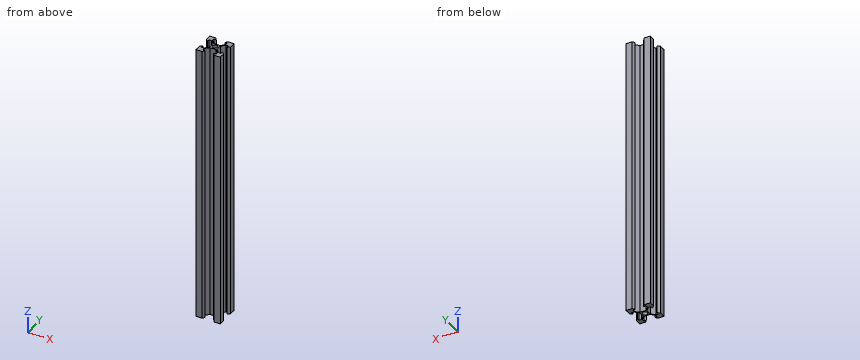
Autodesk Inventor part; units mm, degrees
ref_plane "YZ Plane" through (0, 0, 0) normal (1, 0, 0) x (0, 1, 0)
ref_plane "XZ Plane" through (0, 0, 0) normal (0, 1, 0) x (-1, 0, 0)
ref_plane "XY Plane" through (0, 0, 0) normal (0, 0, 1) x (1, 0, 0)
sketch "Sketch1" plane through (0, 0, 0) normal (0, 0, 1) x (1, 0, 0)
  line L0 (-5, 10) -> (-3.5, 8)
  line L1 (-3.5, 8) -> (-5.5, 8)
  line L2 (5.5, 8) -> (3.5, 8)
  line L3 (3.5, 8) -> (5, 10)
  line L4 (-5.5, 8) -> (-5.5, 6)
  line L5 (5.5, 8) -> (5.5, 6)
  line L6 (-5.5, 6) -> (-2.5, 3)
  line L7 (5.5, 6) -> (2.5, 3)
  line L8 (-2.5, 3) -> (2.5, 3)
  line L9 (-10, 10) -> (-5, 10)
  line L10 (5, 10) -> (10, 10)
  line L11 (3, 2.5) -> (3, -2.5)
  line L12 (3, -2.5) -> (6, -5.5)
  line L13 (6, -5.5) -> (8, -5.5)
  line L14 (8, -5.5) -> (8, -3.5)
  line L15 (8, -3.5) -> (10, -5)
  line L16 (3, 2.5) -> (6, 5.5)
  line L17 (6, 5.5) -> (8, 5.5)
  line L18 (8, 5.5) -> (8, 3.5)
  line L19 (8, 3.5) -> (10, 5)
  line L20 (10, 10) -> (10, 5)
  line L21 (10, -5) -> (10, -10)
  line L22 (-10, 5) -> (-8, 3.5)
  line L23 (-8, 3.5) -> (-8, 5.5)
  line L24 (-8, -5.5) -> (-8, -3.5)
  line L25 (-8, -3.5) -> (-10, -5)
  line L26 (-8, 5.5) -> (-6, 5.5)
  line L27 (-8, -5.5) -> (-6, -5.5)
  line L28 (-6, 5.5) -> (-3, 2.5)
  line L29 (-6, -5.5) -> (-3, -2.5)
  line L30 (-3, 2.5) -> (-3, -2.5)
  line L31 (-10, 10) -> (-10, 5)
  line L32 (-10, -5) -> (-10, -10)
  line L33 (-2.5, -3) -> (2.5, -3)
  line L34 (2.5, -3) -> (5.5, -6)
  line L35 (5.5, -6) -> (5.5, -8)
  line L36 (5.5, -8) -> (3.5, -8)
  line L37 (3.5, -8) -> (5, -10)
  line L38 (-2.5, -3) -> (-5.5, -6)
  line L39 (-5.5, -6) -> (-5.5, -8)
  line L40 (-5.5, -8) -> (-3.5, -8)
  line L41 (-3.5, -8) -> (-5, -10)
  line L42 (-10, -10) -> (-5, -10)
  line L43 (5, -10) -> (10, -10)
  point P0 (0, 0)
  point P1 (0, 0)
  point P2 (0, 0)
  dimension "d0" = 20
  dimension "d1" = 20
  dimension "d3" = 2
  dimension "d4" = 2
  dimension "d6" = 1.5
  dimension "d7" = 2
  dimension "d8" = 2
  dimension "d9" = 3
  dimension "d11" = 3
  dimension "d12" = 3
  dimension "d13" = 5
  dimension "d22" = 5
  dimension "d24" = 3
  dimension "d25" = 3
  dimension "d26" = 2
  dimension "d27" = 5
  dimension "d28" = 2
  dimension "d29" = 2
  dimension "d30" = 1.5
  dimension "d31" = 3
  dimension "d32" = 5
  dimension "d33" = 5
  dimension "d35" = 5
  dimension "d36" = 5
  dimension "d37" = 5
  dimension "d38" = 5
  dimension "d40" = 3
  dimension "d41" = 3
  dimension "d42" = 2
  dimension "d43" = 2
  dimension "d48" = 3
  dimension "d49" = 3
  dimension "d50" = 3
  dimension "d51" = 3
  dimension "d52" = 0.5
  dimension "d53" = 0.5
  dimension "d54" = 0.5
  dimension "d55" = 0.5
  dimension "d56" = 0.5
extrude "Extrusion3" add sketch "Sketch1" along normal blind 230
sketch "Sketch3" plane through (0, 0, 0) normal (0, 0, -1) x (-1, 0, 0)
  circle A0 centre (0, 0) radius 2
  dimension "d59" = 4
extrude "Extrusion4" cut sketch "Sketch3" against normal through all
properties part number "20x20x100 Aluminium VSlot Extrustion"
Geometry: final body of the model. Coordinates: model frame, mm. Coordinates: 2 decimals unless noted, no trailing zeros. Order: outer loops, then holes, each group sorted by start corner. A loop starts at its lowest first (then second) coordinate and runs counter-clockwise, first axis right, second up. Notation, with made-up numbers: M 27,9.25 L 75,9.25 A18 ccw 75,15.25 Z; hole C -35,-35 d2. An arc over 180 degrees is marked long. One line per question, with ' | ' between items. Start each with the question number.
Item 1: Ray query, probe 1 along Y at (x, z) = (0, 129); probe 2 along Y at (x, z) = (-5.25, 33); probe 3 along Y at (x, z) = (6.5, 116). Return the intervals inside material, ascending. Write a range as [from, to].
Item 2: Pin query (flat end, axial travel): pin 1 Ø1.5 at (x, y) = (-0.5, -1.5) entering from +Z; pin 2 Ø6 at (x, z) = (0, 95.5) entering from +Y; pin 3 Ø2.5 at (x, z) = (1, 129.5) entering from -Y; pin 4 Ø5.5 at (x, z) = (-1, 133.5) entering from +Y. Return the tip coordinate at first contact, or that it passes through.
Item 3: Cut plane A-A, the plane x = 0. Return the cut outline in (y, z), then the cut area to 3 significant figures.
A:
1) probe 1: y = [-3, -2], [2, 3] | probe 2: y = [-10, -8], [-5.75, -4.75], [4.75, 5.75], [8, 10] | probe 3: y = [-10, -5.5], [5.5, 10]
2) pin 1: stops at z = 230 | pin 2: stops at y = 3.5 | pin 3: stops at y = -3 | pin 4: stops at y = 8.33
3) outline: M -3,0 L -2,0 L -2,230 L -3,230 Z; M 2,0 L 3,0 L 3,230 L 2,230 Z | area: 460 mm2
